Geometry: final body of the model. Coordinates: model frame, mm. Face numbers are marked on the shaded views. A direction names the side the tool comes from. Give positions to 0.01 mm unless a question says otherwise; leave off trailing zeros. Write each loop counter-clockwise with the first axis right and the second up, starting at its lowest first coordinate (ties: lowest second). Pieces come first, ordered by that corner, then holes.
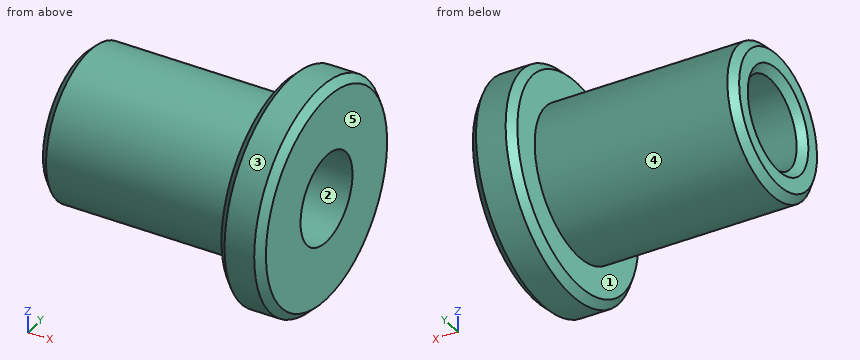
from build123d import *

# Parameters (mm, degrees)
CHANFREIN1_SIZE = 0.5


with BuildPart() as part:
    # Esquisse1 → Base-Révolution (revolve)
    with BuildSketch(Plane.XY, mode=Mode.PRIVATE) as base_r_volution_sk:
        Polygon((0, 3), (0, 5), (13.5, 5), (13.5, 7.5), (16.5, 7.5), (16.5, 3), align=None)
    revolve(base_r_volution_sk.sketch.rotate(Axis((0, 0, 0), (1, 0, 0)), 90), axis=Axis((0, 0, 0), (1, 0, 0)))

    # Chanfrein1
    chanfrein1_edges = [part.edges().sort_by_distance(p)[0] for p in [
        (16.5, 0, -7.5),
        (13.5, 0, -7.5),
        (0, 0, -5),
        (0, 0, -3),
    ]]
    chamfer(chanfrein1_edges, length=CHANFREIN1_SIZE)


solid = part.part
Q1. Ray query, line 1 along Y through (x, z) = (7.5, 0); line 2 along Y through (x, z) = (12.5, -4); line 3 along Y through (x, z) = (13, -2). Return the intervals inside material, ascending.
Filled sheet:
line 1: y = -5 to -3, 3 to 5
line 2: y = -3 to 3
line 3: y = -4.58 to -2.24, 2.24 to 4.58
Q2. Pin query (flat end, axial travel): P1, Ø1.5, axis at y = 4.5, z = 1, coming from the -X side; P2, Ø1, axis at y = 4.5, z = 4.5, coming from the -X side; P3, Ø2, axis at x = 2, y = -2.5, coming from the +Z side. Return the tip coordinate at first contact, or that it passes through.
Filled sheet:
P1: stops at x = 0
P2: stops at x = 13.5
P3: stops at z = 4.77
Q3. Section C-C on x = 5.5. Output: boundary loops of the cut face in (y, z), plus the area to 3 significant figures.
Filled sheet:
outline: circle Ø10 at (0, 0); hole circle Ø6 at (0, 0)
area: 50.3 mm2
Q4. Section A-A on z = 0. Output: boundary loops of the cut face in (x, y).
Filled sheet:
outline: (0, -4.5) - (0.5, -5) - (13.5, -5) - (13.5, -7) - (14, -7.5) - (16, -7.5) - (16.5, -7) - (16.5, -3) - (0.5, -3) - (0, -3.5) - close; (0, 3.5) - (0.5, 3) - (16.5, 3) - (16.5, 7) - (16, 7.5) - (14, 7.5) - (13.5, 7) - (13.5, 5) - (0.5, 5) - (0, 4.5) - close
Q5. Access query for the marked faces 4 and 5. Directions: +Z, -Z, +X, -X, +Y, -Y. A direction counts if a zero-diameter tool reaches every point of the face in a straight line with its end or side. Return the directions, or none.
Filled sheet:
face 4: -X
face 5: +Z, -Z, +X, +Y, -Y
Q6. Pull-direction query (Z, two-part tool) for the marked faces 1, 2 and 3; classes: released by +Z, released by -Z, zero draft, split by the parting line, or undercut.
Filled sheet:
face 1: zero draft
face 2: undercut
face 3: split by the parting line
